The drawing under review shows one solid part. Ordinate dimensions are in mm from its lowest x, y, z. A direction names the side the tool comes from. Coordinates: 2 decimals unless noted, no trailing zeros. Loops run counter-clockwise (first coordinate to the right, second up) from the corner with the lowest first, then second, coordinate; pieces in that order, holes last. Notation, with made-up numbers: (71, -22.5) - (102, -22.5) arc R33 ccw to (102, 10.5) - close; hole circle Ø9 at (31, -25.5). An arc over 180 degrees is marked (long way). Answer as a JSON object with one key per item and string values. Group by question number.
Item 1: We need section C-C (z = 17). Give the boundary of the cut face in (x, y).
Item 2: To check wall thickness, follow line 1 (X direction, y = 60, z = 31); line 2 (Y direction, x = 60, z = 47); line 3 (X direction, y = 60, z = 14). State the ranges of each line that lie inside material, in increasing order.
Item 3: We need section D-D (z = 29). Give the boundary of the cut face in (x, y), then the cut area to 3 significant figures.
Item 4: We need section A-A (x = 60). Give the boundary of the cut face in (y, z).
Item 5: Clearance check with flat-ended pins moving along their axes: pin 1 (10 mm diameter, centred on y = 63.5, z = 33.5, fed in from +X); pin 2 (16.5 mm diameter, centred on x = 59, z = 17.5, fed in from -Y); pin 3 (2 mm diameter, centred on y = 87, z = 24.5, fed in from -X); pin 4 (12 mm diameter, centred on x = 81.5, z = 35.5, fed in from +Y). State where each tip first meets the part, or that it passes through.
Item 6: We need section B-B (y = 60). Give the boundary of the cut face in (x, z), then the cut area to 3 significant figures.
Item 7: Tool access review of the marked faces 5, 6 and 7: name each direction out of +Z, -Z, +X, -X, +Y, -Y from which nothing blocks a thin tool from reaching the whole face with its end or side.
Item 8: Mouldability with a two-part tool opening along Z and no side actions: class the marked faces 1, 2, 3 and 4 as released by +Z, released by -Z, zero draft, split by the parting line, or undercut.
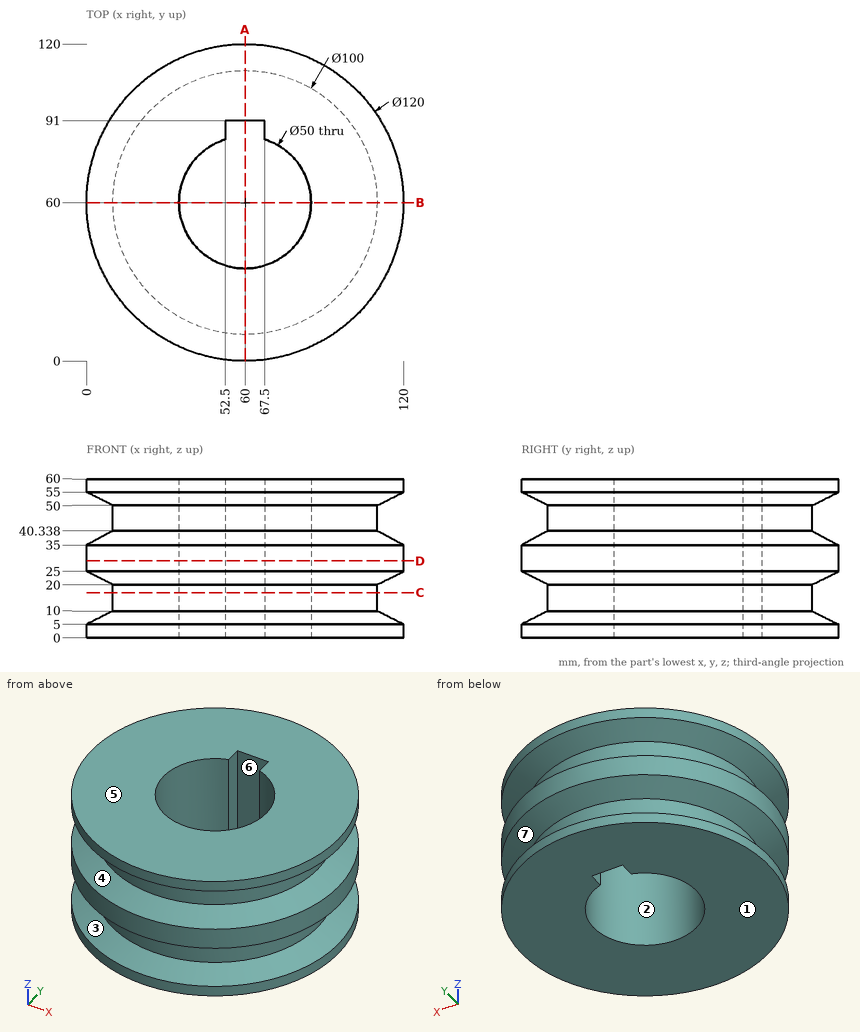
Check sheet entries:
{
 "1": {"outline": "circle Ø100 at (60, 60); hole (52.5, 83.85) arc R25 ccw (long way) to (67.5, 83.85) - (67.5, 91) - (52.5, 91) - close"},
 "2": {"line 1": "x = 0 to 35, 85 to 120", "line 2": "y = 10 to 35, 91 to 110", "line 3": "x = 10 to 35, 85 to 110"},
 "3": {"outline": "circle Ø120 at (60, 60); hole (52.5, 83.85) arc R25 ccw (long way) to (67.5, 83.85) - (67.5, 91) - (52.5, 91) - close", "area": "9,250 mm2"},
 "4": {"outline": "(0, 0) - (35, 0) - (35, 60) - (0, 60) - (0, 55) - (10, 50) - (10, 40.34) - (0, 35) - (0, 25) - (10, 20) - (10, 10) - (0, 5) - close; (91, 0) - (120, 0) - (120, 5) - (110, 10) - (110, 20) - (120, 25) - (120, 35) - (110, 40.34) - (110, 50) - (120, 55) - (120, 60) - (91, 60) - close"},
 "5": {"pin 1": "stops at x = 120", "pin 2": "stops at y = 0", "pin 3": "stops at x = 5.99", "pin 4": "stops at y = 117.96"},
 "6": {"outline": "(0, 0) - (35, 0) - (35, 60) - (0, 60) - (0, 55) - (10, 50) - (10, 40.34) - (0, 35) - (0, 25) - (10, 20) - (10, 10) - (0, 5) - close; (85, 0) - (120, 0) - (120, 5) - (110, 10) - (110, 20) - (120, 25) - (120, 35) - (110, 40.34) - (110, 50) - (120, 55) - (120, 60) - (85, 60) - close", "area": "3,600 mm2"},
 "7": {"face 5": "+Z, +X, -X, +Y, -Y", "face 6": "+Z, -Z", "face 7": "none"},
 "8": {"face 1": "released by -Z", "face 2": "zero draft", "face 3": "undercut", "face 4": "undercut"}
}
